The figure shows three views and two pictorial views of one solid part (mm, origin at its lowest corner). Answer the questions. A direction names the side the tool comes from. Give positions to 0.01 mm unless a question says otherwise; leave off trailing zeros. Write each loop counter-clockwise with the first axis right and the second up, starting at its lowest first coordinate (ties: lowest second). Pieces come first, ordered by that corner, then holes. Notation, with made-up numbers: (66.25, 17.25) -> (108.25, 17.25) arc R16 ccw to (108.25, 35.25) -> close; hole circle Ø9 at (34, 82.5). An arc over 180 degrees is marked (long way). Use a Markdown table: item, result.
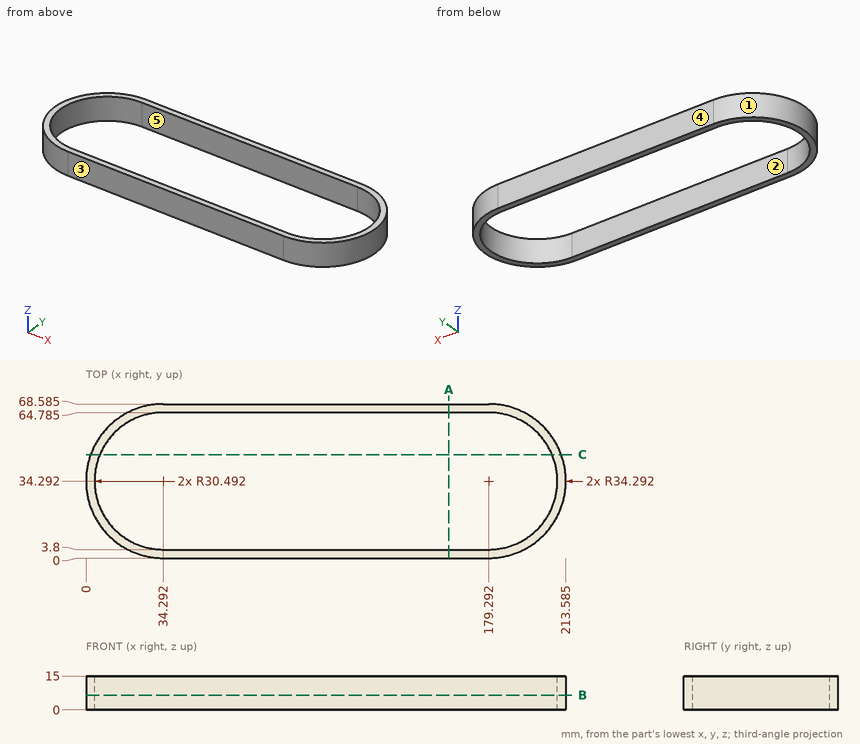
Item 1: For a pull along Y with two mould halves and no side action, classify the marked faces 1, 2 and 3 as +Y half, -Y half, draft (parallel to the pull), parting line (faces both ways), or undercut.
Return value:
| item | result |
|---|---|
| face 1 | parting line |
| face 2 | undercut |
| face 3 | -Y half |
Item 2: A tool of negligible diameter and unlimited length cuts with its end or side. For the marked faces 4 and 5, from which of +Z, -Z, +X, -X, +Y, -Y can it reach the whole face along a straight path? Write none if from no direction.
Return value:
| item | result |
|---|---|
| face 4 | +Z, -Z, +X, -X, +Y |
| face 5 | +Z, -Z |
Item 3: A cutting plane is placed at B-B (z = 6.5). Give the vertices of the cut face in (x, y) (1 decimal).
Return value:
| item | result |
|---|---|
| outline | (34.3, 0) -> (179.3, 0) arc R34.3 ccw to (179.3, 68.6) -> (34.3, 68.6) arc R34.3 ccw to start; hole (34.3, 3.8) -> (179.3, 3.8) arc R30.5 ccw to (179.3, 64.8) -> (34.3, 64.8) arc R30.5 ccw to start |
Item 4: Straight lines are drawn through the part: line 1 along Y through (x, z) = (145.5, 7) (1 decimal); line 2 along X through (y, z) = (33.5, 7.75) (1 decimal); line 3 along X through (y, z) = (54, 7.75) (1 decimal). For each, find the intervals that lie inside material, in ascending order. Write a range as [from, to].
Return value:
| item | result |
|---|---|
| line 1 | [0, 3.8], [64.8, 68.6] |
| line 2 | [0, 3.8], [209.8, 213.6] |
| line 3 | [6.2, 11], [202.6, 207.4] |
Item 5: Each of these flat-tipped pins is pushed along its axis until it touches: P1, Ø4, axis at y = 27, z = 4.5, coming from the -X side; P2, Ø1, axis at y = 61, z = 9, coming from the +X side; P3, Ø6, axis at y = 21.5, z = 3.5, coming from the -X side. Where does it stop, or does it pass through?
Return value:
| item | result |
|---|---|
| P1 | x = 0.41 |
| P2 | x = 201.41 |
| P3 | x = 1.43 |
Item 6: A cutting plane is placed at A-A (x = 161.5). Give the vertices of the cut face in (y, z) (1 decimal), then the cut area to 3 significant figures.
Return value:
| item | result |
|---|---|
| outline | (0, 0) -> (3.8, 0) -> (3.8, 15) -> (0, 15) -> close; (64.8, 0) -> (68.6, 0) -> (68.6, 15) -> (64.8, 15) -> close |
| area | 114 mm^2 |
Item 7: A cutting plane is placed at C-C (y = 46). Give the vertices of the cut face in (x, z) (1 decimal), then the cut area to 3 significant figures.
Return value:
| item | result |
|---|---|
| outline | (2.1, 0) -> (6.1, 0) -> (6.1, 15) -> (2.1, 15) -> close; (207.4, 0) -> (211.5, 0) -> (211.5, 15) -> (207.4, 15) -> close |
| area | 122 mm^2 |
